The listing builds one solid part. Answer for the finished solid, in the listing's coordinates (mm). Face numbers are marked on the shaded views. Coordinates: 2 decimals unless noted, no trailing zeros. Write each loop counter-clockwise with the first axis right and the second up, starting at its lowest first coordinate (ties: lowest second). Pieces come first, ordered by that corner, then holes.
Autodesk Inventor part; units mm, degrees
ref_plane "YZ Plane" through (0, 0, 0) normal (1, 0, 0) x (0, 1, 0)
ref_plane "XZ Plane" through (0, 0, 0) normal (0, 1, 0) x (-1, 0, 0)
ref_plane "XY Plane" through (0, 0, 0) normal (0, 0, 1) x (1, 0, 0)
sketch "Sketch1" plane through (0, 0, 0) normal (0, 0, 1) x (1, 0, 0)
  circle A0 centre (0, 0) radius 39
  dimension "d0" = 78
extrude "Extrusion1" add sketch "Sketch1" along normal blind 484
fillet "Fillet1" radius 25 1 edges at (-39, 0, 484)
fillet "Fillet4" radius 5 1 edges at (-39, 0, 0)
properties part number "Accumulator"
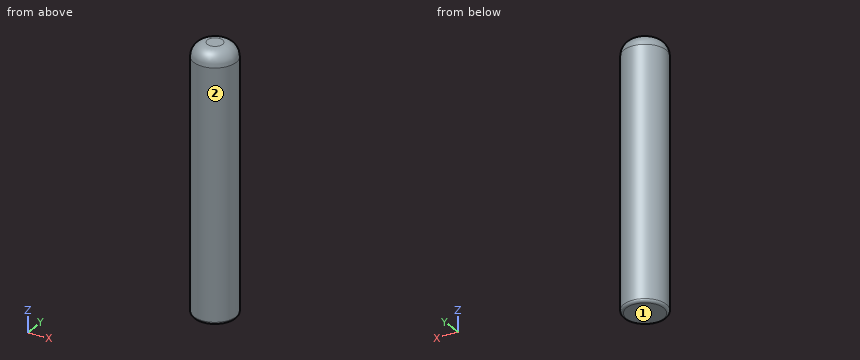
1. Find the intervals of material crossed by L1, parallel to Y at x = 19, z = 168.5; L2, parallel to X at y = -15, z = 114.5; L3, parallel to Y at x = 0.5, z = 433, in increasing order.
Results found:
L1: y = -34.06 to 34.06
L2: x = -36 to 36
L3: y = -39 to 39
2. For a pull along X with two mould halves and no side action, classify the marked faces 1 and 2 as pulls with the +X half, pulls with the -X half, needs draft (parallel to the pull), parting line crosses it, or undercut.
Results found:
face 1: needs draft
face 2: parting line crosses it
3. Flat-ended cylindrical pins translate along their axes: P1, Ø2, axis at x = -19.5, y = 23.5, coming from the -Z side; P2, Ø8, axis at x = -29, z = 333, coming from the -Y side; P3, Ø1, axis at x = -9, y = -30.5, coming from the +Z side; P4, Ø10, axis at x = 0.5, z = 225, coming from the +Y side. Find the tip coordinate at first contact, or state that the pin passes through.
Results found:
P1: stops at z = 0
P2: stops at y = -29.93
P3: stops at z = 477.05
P4: stops at y = 39
4. Section A-A on z = 375 is taken. Give the vertices of the cut face in (x, y), then the cut area to 3 significant figures.
Results found:
outline: circle Ø78 at (0, 0)
area: 4,780 mm2
